Input: part model. Units: mm. Frame: model coordinates. Face numbers are marked on the shaded views. A direction names the side the tool comes from. Coordinates: 2 decimals unless noted, no trailing zeros. Write each loop counter-clockwise with the first axis right and the second up, starting at its lowest first coordinate (ties: lowest second). Pieces come first, ordered by that corner, then holes. Notation, with made-up numbers: (56.25, -13.5) - (94.25, -13.5) arc R19 ccw to (94.25, 6.5) - close; hole circle Ø10 at (10.5, 32.25). An arc over 180 degrees is marked (long way). One line per question, with ' | ' between items. Start each with the question number.
1) Section query D-D on y = 52.5. Return loops of the section in (x, z), and give its area (3 significant figures).
2) Section query C-C on x = 61. Return loops of the section in (y, z), and give its area (3 significant figures).
3) Reachability of the marked faces 1 and 2 from +Z, -Z, +X, -X, +Y, -Y: full face, straight path, thin tool, end or side. Return the list, or none.
4) Section query A-A on x = 51. Return loops of the section in (y, z), and give its area (3 significant figures).
5) Section query B-B on x = 24. Return loops of the section in (y, z), and give its area (3 significant figures).
6) First-contact query: P1, Ø1.3, axis at y = 42.5, z = 6.5, coming from the +X side; P2, Ø3.5, axis at x = 7.96, y = 7.61, coming from the +Z side. Flat tips, straight axial feed; report the tip coordinate or a pass-through.
7) Line query: line 1 (Y direction, x = 52, z = 4.5); line 2 (Y direction, x = 34.5, z = 8); line 3 (X direction, y = 9, z = 7.75). Output: solid intervals per line, ascending.
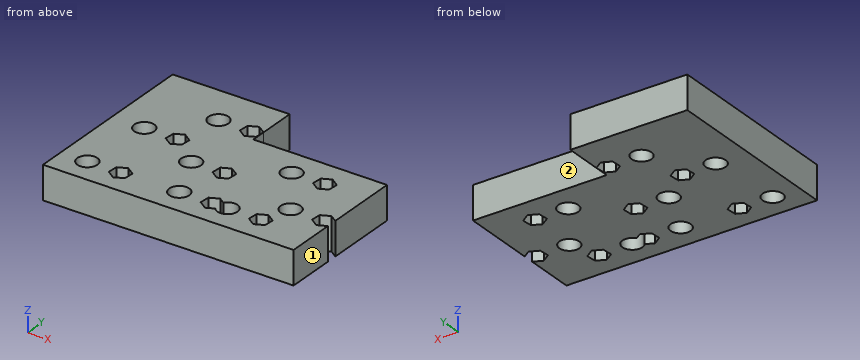
```python
from build123d import *

# Parameters (mm, degrees)
BOSS_EXTRUDE1_DEPTH       = 10
SKETCH2_R                 = 3
CUT_EXTRUDE1_DEPTH        = 10
SKETCH_PATTERN1_OUTLINE_R = 3
SKETCH_PATTERN1_DEPTH     = 10


# Read off the part's stored shape, not the designer's step: Sketch-Pattern1
with BuildPart() as part:
    # Sketch1 → Boss-Extrude1 (new body)
    with BuildSketch(Plane.XY):
        Polygon((0, 0), (75, 0), (75, 40), (35, 40), (35, 55.537974684), (0, 55.537974684), align=None)
    extrude(amount=BOSS_EXTRUDE1_DEPTH)

    # Sketch2 → Cut-Extrude1 (cut)
    with BuildSketch(Plane.XY.offset(10)):
        with Locations((7.962950949, 7.607986586)):
            Circle(SKETCH2_R)
        Polygon((20.345287783, 5.925870596), (20.586453467, 8.872391359), (18.155274475, 10.55450735), (15.482929799, 9.290102577), (15.241764115, 6.343581814), (17.672943107, 4.661465823), align=None)
    extrude(amount=-CUT_EXTRUDE1_DEPTH, mode=Mode.SUBTRACT)

    # Sketch-Pattern1 outline → Sketch-Pattern1 (cut)
    with BuildSketch(Plane.XY):
        with Locations((9.737115818, 29.458094158)):
            Circle(SKETCH_PATTERN1_OUTLINE_R)
        with Locations((52.327690787, 31.62602284)):
            Circle(SKETCH_PATTERN1_OUTLINE_R)
        Polygon((36.229757623, 20.763839411), (38.660936615, 19.08172342), (41.333281291, 20.346128193), (41.574446975, 23.292648956), (39.143267983, 24.974764947), (36.470923307, 23.710360174), align=None)
        with Locations((28.950944457, 22.028244183)):
            Circle(SKETCH_PATTERN1_OUTLINE_R)
        Polygon((35, 44.312366767), (35, 44.387559798), (32.574645536, 46.065645838), (29.90230086, 44.801241065), (29.661135176, 41.854720302), (32.092314168, 40.172604311), (34.764658844, 41.437009084), align=None)
        with Locations((22.38232201, 43.119125074)):
            Circle(SKETCH_PATTERN1_OUTLINE_R)
        Polygon((17.015928983, 28.193689386), (19.447107975, 26.511573395), (22.119452651, 27.775978168), (22.360618335, 30.722498931), (19.929439343, 32.404614922), (17.257094667, 31.140210149), align=None)
        Polygon((59.606503953, 30.361618067), (62.037682945, 28.679502076), (64.710027621, 29.943906849), (64.951193305, 32.890427612), (62.520014313, 34.572543603), (59.847669637, 33.30813883), align=None)
        with Locations((62.661508703, 16.393274831)):
            Circle(SKETCH_PATTERN1_OUTLINE_R)
        Polygon((69.940321868, 15.128870058), (72.37150086, 13.446754067), (75, 14.690413573), (75, 17.854876903), (72.853832228, 19.339795594), (70.181487552, 18.075390822), align=None)
        with Locations((35.250227337, 7.942687663)):
            Circle(SKETCH_PATTERN1_OUTLINE_R)
        Polygon((56.966278334, 6.67828289), (59.397457326, 4.996166899), (62.069802002, 6.260571672), (62.310967686, 9.207092435), (59.879788694, 10.889208426), (57.207444018, 9.624803653), align=None)
        with BuildLine():
            Line((44.960219495, 4.996166899), (47.312866175, 6.109308373))
            ThreePointArc((47.312866175, 6.109308373), (52.686542056, 8.017104238), (47.224860539, 9.656040644))
            Line((47.224860539, 9.656040644), (45.442550863, 10.889208426))
            Line((45.442550863, 10.889208426), (42.770206187, 9.624803653))
            Line((42.770206187, 9.624803653), (42.529040503, 6.67828289))
            Line((42.529040503, 6.67828289), (44.960219495, 4.996166899))
        make_face()
    extrude(amount=SKETCH_PATTERN1_DEPTH, mode=Mode.SUBTRACT)


solid = part.part
```
Answer key:
1) outline: (0, 0) - (35, 0) - (35, 10) - (0, 10) - close | area: 350 mm²
2) outline: (0, 0) - (5.75, 0) - (5.75, 10) - (0, 10) - close; (10.11, 0) - (13.9, 0) - (13.9, 10) - (10.11, 10) - close; (18.89, 0) - (29.4, 0) - (29.4, 10) - (18.89, 10) - close; (33.85, 0) - (40, 0) - (40, 10) - (33.85, 10) - close | area: 262 mm²
3) face 1: +Z, -Z, +X, +Y, -Y | face 2: +Z, -Z, +X, +Y
4) outline: (0, 0) - (5.25, 0) - (5.25, 10) - (0, 10) - close; (10.64, 0) - (28.94, 0) - (28.94, 10) - (10.64, 10) - close; (34.32, 0) - (40, 0) - (40, 10) - (34.32, 10) - close | area: 292 mm²
5) outline: (0, 0) - (40.59, 0) - (40.59, 10) - (0, 10) - close; (45.65, 0) - (55.54, 0) - (55.54, 10) - (45.65, 10) - close | area: 505 mm²
6) P1: x = 35 | P2: through
7) line 1: 0 to 6.03, 9.85 to 28.64, 34.61 to 40 | line 2: 0 to 5.04, 10.85 to 41.31, 44.73 to 55.54 | line 3: 0 to 5.31, 10.62 to 15.46, 20.4 to 32.44, 38.06 to 42.72, 52.49 to 57.16, 62.29 to 75
